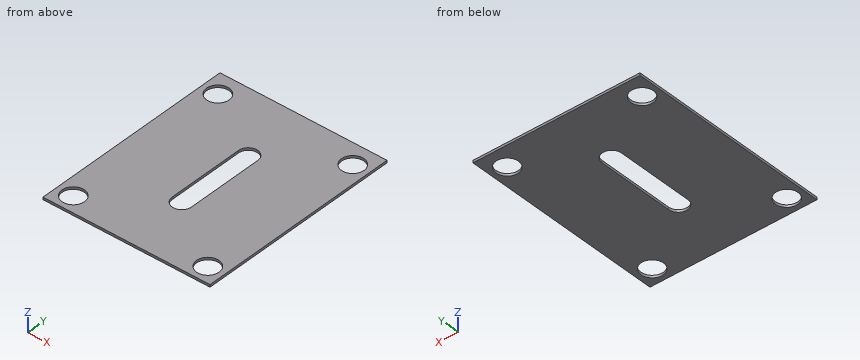
```python
from build123d import *

# Parameters (mm, degrees)
SKETCH1_W           = 41.4
SKETCH1_H           = 50.8
BOSS_EXTRUDE1_DEPTH = 0.6096
CUT_EXTRUDE2_DEPTH  = 0.6096
SKETCH9_R           = 2.794
CUT_EXTRUDE3_DEPTH  = 0.6096


with BuildPart() as part:
    # Sketch1 → Boss-Extrude1 (new body)
    with BuildSketch(Plane.XY):
        with Locations((-4635.961935484, -4371.258064516)):
            Rectangle(SKETCH1_W, SKETCH1_H)
    extrude(amount=BOSS_EXTRUDE1_DEPTH)

    # Sketch4 → Cut-Extrude2 (cut)
    with BuildSketch(Plane.XY.offset(0.6096)):
        with BuildLine():
            Line((-4638.343185484, -4380.783064516), (-4638.343185484, -4361.733064516))
            ThreePointArc((-4638.343185484, -4361.733064516), (-4635.961935484, -4359.351814516), (-4633.580685484, -4361.733064516))
            Line((-4633.580685484, -4361.733064516), (-4633.580685484, -4380.783064516))
            ThreePointArc((-4633.580685484, -4380.783064516), (-4635.961935484, -4383.164314516), (-4638.343185484, -4380.783064516))
        make_face()
    extrude(amount=-CUT_EXTRUDE2_DEPTH, mode=Mode.SUBTRACT)

    # Sketch9 → Cut-Extrude3 (cut)
    with BuildSketch(Plane(origin=(0, 0, 0), x_dir=(-1, 0, 0), z_dir=(0, 0, -1))):
        with Locations((4619.267234292, -4351.044101977)):
            Circle(SKETCH9_R)
        with Locations((4652.667204287, -4351.088871634)):
            Circle(SKETCH9_R)
        with Locations((4619.28588452, -4392.63411548)):
            Circle(SKETCH9_R)
        with Locations((4652.637986448, -4392.63411548)):
            Circle(SKETCH9_R)
    extrude(amount=-CUT_EXTRUDE3_DEPTH, mode=Mode.SUBTRACT)


solid = part.part
```
Model file for the job. Use its own axes, mm. Coordinates: 2 decimals unless noted, no trailing zeros. Order: outer loops, then holes, each group sorted by start corner. A loop starts at its lowest first (then second) coordinate and runs counter-clockwise, first axis right, second up. Notation, with made-up numbers: M 17,57 L 70,57 A22 cw 70,69 Z; hole C -38.75,73 d9. An arc over 180 degrees is marked long. Answer as CSV lines item,"result".
(1) Flat gauge pins, fed straight in: pin 1 (7.5 mm diameter, centred on x = -4652.64, y = -4392.63, fed in from +Z); pin 2 (5 mm diameter, centred on x = -4652.67, y = -4351.09, fed in from -Z). Where does each tip first touch, or does it go through?
Geometry says:
pin 1,"stops at z = 0.61"
pin 2,"passes through"
(2) Wall check: line 1 along Y through (x, z) = (-4621, 0.35); line 2 along Y through (x, z) = (-4652, 0.3); line 3 along X through (y, z) = (-4373, 0.2). Give the ranges that are in metal, low to high.
Geometry says:
line 1,"y = -4396.66 to -4394.84, -4390.43 to -4353.24, -4348.85 to -4345.86"
line 2,"y = -4396.66 to -4395.35, -4389.91 to -4353.8, -4348.38 to -4345.86"
line 3,"x = -4656.66 to -4638.34, -4633.58 to -4615.26"
(3) Band-saw the part on B-B, the plane x = -4652.5. List the corners of the cut face in (y, z), then the cut area to 3 significant figures.
Geometry says:
outline,"M -4396.66,0 L -4395.42,0 L -4395.42,0.61 L -4396.66,0.61 Z; M -4389.84,0 L -4353.88,0 L -4353.88,0.61 L -4389.84,0.61 Z; M -4348.3,0 L -4345.86,0 L -4345.86,0.61 L -4348.3,0.61 Z"
area,"24.2 mm2"
(4) Band-saw the part on A-A, the plane y = -4379. List the corners of the cut face in (x, z), then the cut area to 3 significant figures.
Geometry says:
outline,"M -4656.66,0 L -4638.34,0 L -4638.34,0.61 L -4656.66,0.61 Z; M -4633.58,0 L -4615.26,0 L -4615.26,0.61 L -4633.58,0.61 Z"
area,"22.3 mm2"
(5) Band-saw the part on D-D, the plane x = -4621. List the corners of the cut face in (y, z).
Geometry says:
outline,"M -4396.66,0 L -4394.84,0 L -4394.84,0.61 L -4396.66,0.61 Z; M -4390.43,0 L -4353.24,0 L -4353.24,0.61 L -4390.43,0.61 Z; M -4348.85,0 L -4345.86,0 L -4345.86,0.61 L -4348.85,0.61 Z"
(6) Band-saw the part on C-C, the plane z = 0.15. List the corners of the cut face in (x, y), then the cut area to 3 significant figures.
Geometry says:
outline,"M -4656.66,-4396.66 L -4615.26,-4396.66 L -4615.26,-4345.86 L -4656.66,-4345.86 Z; hole C -4652.67,-4351.09 d5.59; hole C -4652.64,-4392.63 d5.59; hole M -4638.34,-4380.78 A2.38 ccw -4633.58,-4380.78 L -4633.58,-4361.73 A2.38 ccw -4638.34,-4361.73 Z; hole C -4619.29,-4392.63 d5.59; hole C -4619.27,-4351.04 d5.59"
area,"1,900 mm2"
